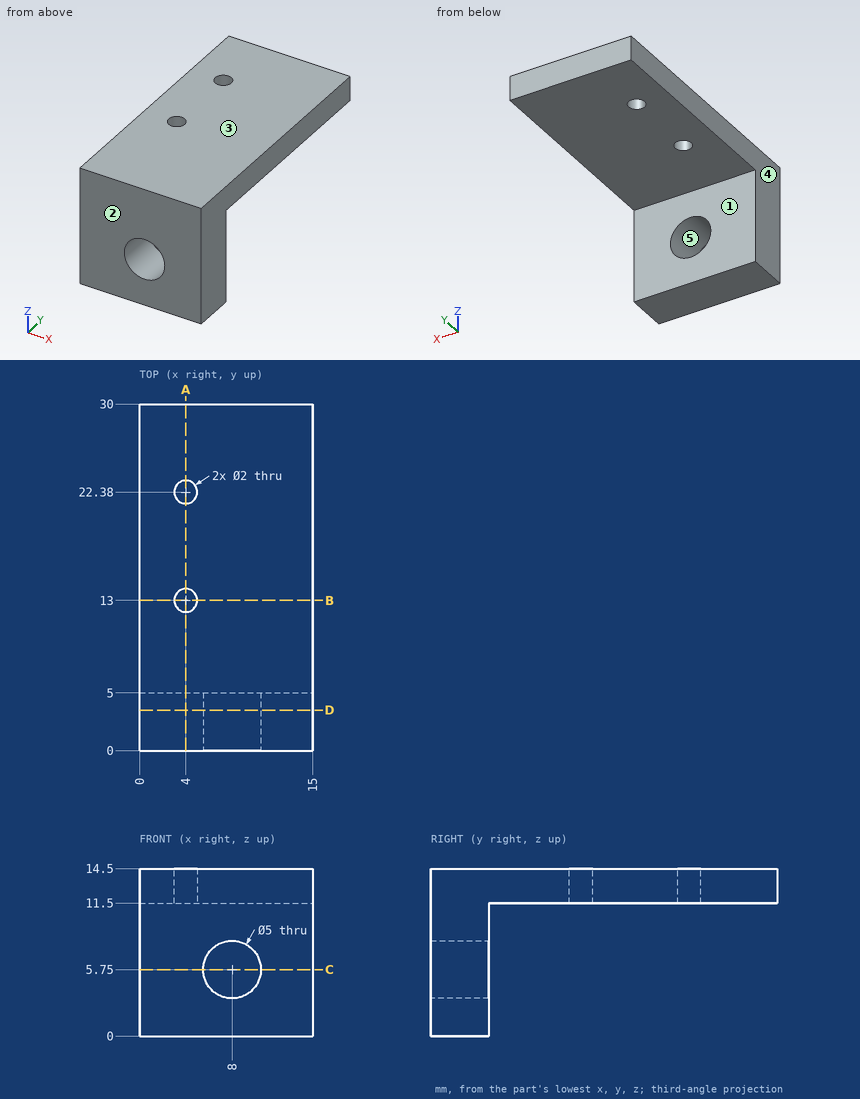
Design review of the part shown in the three views and the two pictorial views. Dimensions are in mm from the part's minimum x, y and z. A direction names the side the tool comes from. Give positions to 0.01 mm unless a question says otherwise; leave off trailing zeros. Write each loop counter-clockwise with the first axis right and the second up, starting at its lowest first coordinate (ties: lowest second). Pieces come first, ordered by that corner, then holes.
(1) Add section C-C (z = 5.75). Give the boundary of the cut face in (x, y).
Checked values:
outline: (0, 0) - (5.5, 0) - (5.5, 5) - (0, 5) - close; (10.5, 0) - (15, 0) - (15, 5) - (10.5, 5) - close
(2) Clearance check with flat-ended pins moving along their axes: pin 1 Ø8 at (x, z) = (8, 5.75) entering from +Y; pin 2 Ø2 at (x, z) = (13.5, 12) entering from -Y. State where each tip first meets the part, or that it passes through.
Checked values:
pin 1: stops at y = 5
pin 2: stops at y = 0
(3) Tool access review of the marked faces 1 and 2: name each direction out of +Z, -Z, +X, -X, +Y, -Y from which nothing blocks a thin tool from reaching the whole face with its end or side.
Checked values:
face 1: -Z, +X, -X, +Y
face 2: +Z, -Z, +X, -X, -Y
(4) Wall thickness on line 1 along Y through (x, z) = (4, 12.35); line 2 along X through (y, z) = (2.45, 5.75); line 3 along Z through (x, y) = (7, 16.75): over which ranges is each line inside the solid? List them lowest first.
Checked values:
line 1: y = 0 to 12, 14 to 21.38, 23.38 to 30
line 2: x = 0 to 5.5, 10.5 to 15
line 3: z = 11.5 to 14.5
(5) Add section D-D (y = 3.5). Give the boundary of the cut face in (x, z).
Checked values:
outline: (0, 0) - (15, 0) - (15, 14.5) - (0, 14.5) - close; hole circle Ø5 at (8, 5.75)
(6) Add section A-A (x = 4). Give the boundary of the cut face in (y, z), and give its area (4 significant figures).
Checked values:
outline: (0, 0) - (5, 0) - (5, 11.5) - (12, 11.5) - (12, 14.5) - (0, 14.5) - close; (14, 11.5) - (21.38, 11.5) - (21.38, 14.5) - (14, 14.5) - close; (23.38, 11.5) - (30, 11.5) - (30, 14.5) - (23.38, 14.5) - close
area: 135.5 mm2
(7) Mouldability with a two-part tool opening along X and no side actions: class the marked faces 3, 4 and 5 as +X half, -X half, draft (parallel to the pull), parting line (faces both ways), or undercut.
Checked values:
face 3: draft
face 4: -X half
face 5: undercut
(8) Add section B-B (y = 13). Give the boundary of the cut face in (x, z).
Checked values:
outline: (0, 11.5) - (3, 11.5) - (3, 14.5) - (0, 14.5) - close; (5, 11.5) - (15, 11.5) - (15, 14.5) - (5, 14.5) - close
